```python
from build123d import *

# Parameters (mm, degrees)
SKETCH1_R                 = 7.5
BOSS_EXTRUDE1_DEPTH       = 20.05
SKETCH3_W                 = 5
SKETCH3_H                 = 5
CUT_EXTRUDE1_DEPTH        = 21
SKETCH6_R                 = 8.5
BOSS_EXTRUDE2_DEPTH       = 24
SKETCH7_R                 = 11.25
BOSS_EXTRUDE3_DEPTH       = 5
SKETCH8_R                 = 30
BOSS_EXTRUDE4_DEPTH       = 5
FILLET1_R                 = 0.6
FILLET2_R                 = 5
M4_CLEARANCE_HOLE1_D      = 4.5
F_1_0MM_DOWEL_HOLE1_D     = 8.255
F_1_0MM_DOWEL_HOLE1_DEPTH = 8
SKETCH13_R                = 7.5
CUT_EXTRUDE2_DEPTH        = 2
M6_CLEARANCE_HOLE1_D      = 6.6
M6_CLEARANCE_HOLE1_DEPTH  = 12


with BuildPart() as part:
    # Sketch1 → Boss-Extrude1 (new body)
    with BuildSketch(Plane.XY):
        Circle(SKETCH1_R)
    extrude(amount=BOSS_EXTRUDE1_DEPTH)

    # Sketch3 → Cut-Extrude1 (cut)
    with BuildSketch(Plane(origin=(0, 0, 0), x_dir=(-1, 0, 0), z_dir=(0, 0, -1))):
        with Locations((0, 7.5)):
            Rectangle(SKETCH3_W, SKETCH3_H)
    extrude(amount=-CUT_EXTRUDE1_DEPTH, mode=Mode.SUBTRACT)

    # Sketch6 → Boss-Extrude2 (add)
    with BuildSketch(Plane.XY.offset(20.05)):
        Circle(SKETCH6_R)
    extrude(amount=BOSS_EXTRUDE2_DEPTH)

    # Sketch7 → Boss-Extrude3 (add)
    with BuildSketch(Plane.XY.offset(44.05)):
        Circle(SKETCH7_R)
    extrude(amount=BOSS_EXTRUDE3_DEPTH)

    # Sketch8 → Boss-Extrude4 (add)
    with BuildSketch(Plane.XY.offset(49.05)):
        Circle(SKETCH8_R)
    extrude(amount=BOSS_EXTRUDE4_DEPTH)

    # Fillet1
    fillet1_edges = [part.edges().sort_by_distance(p)[0] for p in [
        (-8.5, 0, 44.05),
    ]]
    fillet(fillet1_edges, radius=FILLET1_R)

    # Fillet2
    fillet2_edges = [part.edges().sort_by_distance(p)[0] for p in [
        (-11.25, 0, 49.05),
    ]]
    fillet(fillet2_edges, radius=FILLET2_R - 0.0001)  # a hair under: the kernel refuses the full size

    # M4 Clearance Hole1 (through all)
    with Locations(Plane.XY.offset(54.05)):
        with Locations((0, 24), (0, -24), (24, 0), (-24, 0)):
            Hole(M4_CLEARANCE_HOLE1_D / 2)

    # Ø1.0mm Dowel Hole1
    with Locations(Plane(origin=(0, 0, 0), x_dir=(-1, 0, 0), z_dir=(0, 0, -1))):
        with Locations((0, 0)):
            Hole(F_1_0MM_DOWEL_HOLE1_D / 2, depth=F_1_0MM_DOWEL_HOLE1_DEPTH)

    # Sketch13 → Cut-Extrude2 (cut)
    with BuildSketch(Plane(origin=(0, 0, 0), x_dir=(-1, 0, 0), z_dir=(0, 0, -1))):
        Circle(SKETCH13_R)
    extrude(amount=-CUT_EXTRUDE2_DEPTH, mode=Mode.SUBTRACT)

    # M6 Clearance Hole1
    with Locations(Plane(origin=(0, 0, 8), x_dir=(-1, 0, 0), z_dir=(0, 0, -1))):
        with Locations((0, 0)):
            Hole(M6_CLEARANCE_HOLE1_D / 2, depth=M6_CLEARANCE_HOLE1_DEPTH)


solid = part.part
```
Part model, mm, in its own coordinate system. A direction names the side the tool comes from. Round coordinates to 2 decimals unless told otherwise and drop trailing zeros. Loops run counter-clockwise (first coordinate to the right, second up) from the corner with the lowest first, then second, coordinate; pieces in that order, holes last.
Item 1: Cut at C-C, the plane x = 0. State how many separate pieces and enclosed holes the cut face has, then the cut area to 3 significant figures.
Item 2: Cut at A-A, the plane y = -24. Give the cut face in (x, z), then the cut area to 4 significant figures.
Item 3: 3-axis set-ups, long thin cutter, end or side, ignore diameter. For faces 1 (the face through (4.57, 7.167, 31.586)), 2 (the face through (0.488, 21.804, 51.515)), 3 (the face through (0, 5, 11)): which of +Z, -Z, +X, -X, +Y, -Y reach the whole face in a straight line?
Item 4: Mould opens along Y. For faces 4 (the face through (-29.97, 1.32, 51.52)), 5 (the face through (0, 0, 54.05)), 6 (the face through (0.488, -26.196, 51.515)) say: +Y half, -Y half, draft (parallel to the pull), parting line (faces both ways), or undercut.
Item 5: Drill centre lines: line 1 (Y direction, x = 0, z = 50.3); line 2 (Z direction, x = 11, y = -20); line 3 (Y direction, x = -4, z = 16.5). Where is each one in solid material? Low to high.
Item 6: Drop flat-ended pins along their axis: P1, Ø5.5, axis at x = -0.5, z = 12, coming from the +Y side; P2, Ø7.5, axis at x = -1, y = 1, coming from the -Z side; P3, Ø0.6, axis at y = 6.5, z = 11.5, coming from the -X side; P4, Ø10, axis at x = -11, z = 20, coming from the -Y side. Give the stop position or say it passes through.
A:
1. separate pieces: 3
1. enclosed holes: 0
1. area: 883 mm2
2. outline: (-18, 49.05) - (-2.25, 49.05) - (-2.25, 54.05) - (-18, 54.05) - close; (2.25, 49.05) - (18, 49.05) - (18, 54.05) - (2.25, 54.05) - close
2. area: 157.5 mm2
3. face 1: -Z
3. face 2: +Z, -Z
3. face 3: -Z, +Y
4. face 4: parting line
4. face 5: draft
4. face 6: undercut
5. line 1: y = -30 to -26.25, -21.75 to 21.75, 26.25 to 30
5. line 2: z = 49.05 to 54.05
5. line 3: y = -6.34 to 6.34
6. P1: stops at y = 7.07
6. P2: stops at z = 2
6. P3: stops at x = -4.22
6. P4: stops at y = -6.02
